Verification items for the finished model (mm, model axes). Give positions to 0.01 mm unless a question says otherwise; leave off trailing zeros. Write each loop counter-clockwise with the first axis right and the second up, starting at its lowest first coordinate (ties: lowest second). Pieces come first, ordered by that corner, then holes. Notation, with made-up numbers: (-12, 28) -> (-6, 28) arc R26 cw to (-6, 47) -> close; hole circle Ø1 at (-10.75, 52). An arc over 180 degrees is marked (long way). Use one line per item in the form item = value. Start each with the question number.
(1) Section check D-D, the plane z = 8. Record the cut outline in (x, y), plus the area to 3 significant figures.
(2) Section check C-C, the plane x = 0. Record the cut outline in (y, z) (3 decimals), plus the area to 3 significant figures.
(3) Section check A-A, the plane x = -2. Record the cut outline in (y, z).
(4) Section check B-B, the plane y = 0. Record the cut outline in (x, z).
(5) Depth check by flat-ended pin: pin 1 Ø6 at (x, z) = (-2.5, 0) entering from +Y. Enter the tip coordinate at first touch or a pass-through.
(6) Scan lines: L1, parallel to Z at x = 0, y = 3.35 (3 decimals); L2, parallel to Y at x = 0, z = -1; L3, parallel to X at y = 0.25, z = 8.75. Record each from-to range of solid material in increasing order.
(7) Release check for a two-part mould opening along X. For faces 1 (the face through (0.64, 3.87, 5)), 2 (the face through (-3, -1, -9)), 3 (the face through (-0.303, 3.875, -1.886)), 4 (the face through (2.58, -4.97, 1.4)) record: pulls with the +X half, pulls with the -X half, needs draft (parallel to the pull), parting line crosses it, or undercut.
from build123d import *

# Parameters (mm, degrees)
SKETCH1_R                = 5.6
SKETCH1_R_2              = 2.6
BOSS_EXTRUDE1_DEPTH      = 11.508
BOSS_EXTRUDE1_DEPTH_BACK = 9
SKETCH3_R                = 1.397
CUT_EXTRUDE2_DEPTH       = 6.6


with BuildPart() as part:
    # Sketch1 → Boss-Extrude1 (new body, two sides)
    with BuildSketch(Plane.XY) as boss_extrude1_sk:
        Circle(SKETCH1_R)
        Circle(SKETCH1_R_2, mode=Mode.SUBTRACT)
    extrude(amount=BOSS_EXTRUDE1_DEPTH)
    extrude(boss_extrude1_sk.sketch, amount=-BOSS_EXTRUDE1_DEPTH_BACK)

    # Sketch3 → Cut-Extrude2 (cut, through all)
    with BuildSketch(Plane(origin=(0, 0, 0), x_dir=(1, 0, 0), z_dir=(0, 1, 0))):
        with Locations((0, -3.758)):
            Circle(SKETCH3_R)
        with Locations((0, 3.25)):
            Circle(SKETCH3_R)
    extrude(amount=CUT_EXTRUDE2_DEPTH, mode=Mode.SUBTRACT)


solid = part.part
Completed:
q1.outline = circle Ø11.2 at (0, 0); hole circle Ø5.2 at (0, 0)
q1.area = 77.3 mm²
q2.outline = (-5.6, -9) -> (-2.6, -9) -> (-2.6, 11.508) -> (-5.6, 11.508) -> close; (2.6, -9) -> (5.6, -9) -> (5.6, -4.647) -> (2.6, -4.647) -> close; (2.6, -1.853) -> (5.6, -1.853) -> (5.6, 2.361) -> (2.6, 2.361) -> close; (2.6, 5.155) -> (5.6, 5.155) -> (5.6, 11.508) -> (2.6, 11.508) -> close
q2.area = 106 mm²
q3.outline = (-5.23, -9) -> (-1.66, -9) -> (-1.66, 11.51) -> (-5.23, 11.51) -> close; (1.66, -9) -> (5.23, -9) -> (5.23, 11.51) -> (1.66, 11.51) -> close
q4.outline = (-5.6, -9) -> (-2.6, -9) -> (-2.6, 11.51) -> (-5.6, 11.51) -> close; (2.6, -9) -> (5.6, -9) -> (5.6, 11.51) -> (2.6, 11.51) -> close
q5.pin_1 = 5.6
q6.L1 = -9 to -4.647, -1.853 to 2.361, 5.155 to 11.508
q6.L2 = -5.6 to -2.6, 2.6 to 5.6
q6.L3 = -5.59 to -2.59, 2.59 to 5.59
q7.face_1 = undercut
q7.face_2 = needs draft
q7.face_3 = undercut
q7.face_4 = parting line crosses it
